Part model, mm, in its own coordinate system. Face numbers are marked on the shaded views. A direction names the side the tool comes from. Round coordinates to 2 decimals unless told otherwise and drop trailing zeros. Loops run counter-clockwise (first coordinate to the right, second up) from the corner with the lowest first, then second, coordinate; pieces in that order, holes last. Notation, with made-up numbers: (1.25, -40) - (41.25, -40) arc R30 ccw to (41.25, -7) - close; hole circle Ø2 at (39, 66.5). An arc over 180 degrees is marked (long way). Put each result on its own line as item: value.
from build123d import *

# Parameters (mm, degrees)
F0_W     = 109.0900748968
F0_H     = 75.3747150302
F1_DEPTH = 25.4
F2_W     = 43.9951886518
F2_H     = 41.4347245544
F4_R     = 19.656837966
F5_DEPTH = 25.4


with BuildPart() as f1:
    # F0 (on Top) → F1 (new body)
    with BuildSketch(Plane.XY):
        Rectangle(F0_W, F0_H)
    extrude(amount=F1_DEPTH)

    # F2 (on Front) → F3 (revolve)
    with BuildSketch(Plane.XZ):
        with Locations((-21.9975943259, 46.1173622772)):
            Rectangle(F2_W, F2_H)
    revolve(axis=Axis((0, 0, 46.1173622772), (0, 0, -1)))

    # F4 (on face) → F5 (cut)
    with BuildSketch(Plane.XY.offset(66.8347245544)):
        Circle(F4_R)
    extrude(amount=-F5_DEPTH, mode=Mode.SUBTRACT)


solid = f1.part
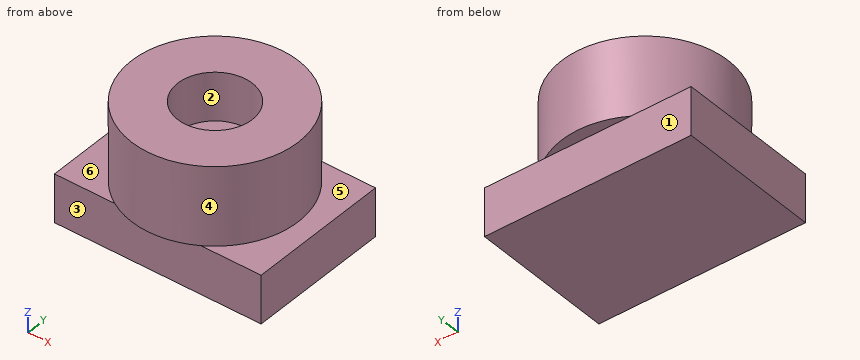
1. Band-saw the part on B-B (z = 50). List the corners of the cut face in (x, y).
A:
outline: circle Ø87.99 at (0, 0); hole circle Ø39.31 at (0, 0)
2. Tool access for the marked faces 4, 5 and 6: list every direction of +Z, -Z, +X, -X, +Y, -Y with a clear straight run to the whole face (end or side of a thin tool).
A:
face 4: +Z
face 5: +Z, +X
face 6: +Z, -X
3. Two-plate mould, pull along Y, no slides. Class the marked faces 1, 2 and 3: pulls with the +Y half, pulls with the -Y half, needs draft (parallel to the pull), parting line crosses it, or undercut.
A:
face 1: pulls with the +Y half
face 2: undercut
face 3: pulls with the -Y half
4. Probe line 1 along Y through (x, z) = (0, 50); line 2 along Z through (x, y) = (-45, -33); line 3 along Y through (x, z) = (11, 6.5). List the from-to ranges inside material, lowest first. Write a range as [from, to].
A:
line 1: y = [-44, -19.66], [19.66, 44]
line 2: z = [0, 25.4]
line 3: y = [-37.69, 37.69]
5. Band-saw the part on C-C (x = -26). List the corners of the cut face in (y, z).
A:
outline: (-37.69, 0) - (37.69, 0) - (37.69, 25.4) - (35.49, 25.4) - (35.49, 66.83) - (-35.49, 66.83) - (-35.49, 25.4) - (-37.69, 25.4) - close
6. Pin check, flat tips, straight feed: P1, Ø1.5, axis at y = -1.5, z = 30, coming from the +X side; P2, Ø12, axis at x = 37.5, z = 32.5, coming from the +Y side; P3, Ø5, axis at y = 6.5, z = 28.5, coming from the +X side. Stop position of each tip, or through.
A:
P1: stops at x = 43.99
P2: stops at y = 30.71
P3: stops at x = 43.81
7. Band-saw the part on A-A (y = 0). List the corners of the cut face in (x, z).
A:
outline: (-54.55, 0) - (54.55, 0) - (54.55, 25.4) - (44, 25.4) - (44, 66.83) - (19.66, 66.83) - (19.66, 41.43) - (-19.66, 41.43) - (-19.66, 66.83) - (-44, 66.83) - (-44, 25.4) - (-54.55, 25.4) - close
8. Band-saw the part on D-D (z = 23). List the corners of the cut face in (x, y).
A:
outline: (-54.55, -37.69) - (54.55, -37.69) - (54.55, 37.69) - (-54.55, 37.69) - close
